Read the model definition and answer for the solid it produces. Units are mm, in the model's axes. Face numbers are marked on the shaded views. A direction names the side the tool comes from. Coordinates: 2 decimals unless noted, no trailing zeros. Write each loop counter-clockwise with the first axis right and the second up, starting at its lowest first coordinate (ties: lowest second). Pieces come first, ordered by that corner, then holes.
(1) Which of the six approach directions +Z, -Z, +X, -X, +Y, -Y give full straight-line access (tool end or side, diameter ignored) to the marked faces 5, 6, 7 and 8?
(2) The part is cut by section A-A, the plane z = 0. Determine the outline of the cut face in (x, y).
(3) The part is cut by section B-B, the plane x = 5. Determine the outline of the cut face in (y, z).
(4) Determine the mould class of the marked faces 1, 2, 3 and 4 for opening direction X: pulls with the +X half, pulls with the -X half, needs draft (parallel to the pull), parting line crosses it, or undercut.
(5) The part is cut by section D-D, the plane z = -2.75. Determine the outline of the cut face in (x, y).
(6) Given pin 1 (1.5 mm diameter, centred on x = 5, z = 0, fed in from -Y) (1 decimal); pin 2 (1.5 mm diameter, centred on x = 9, y = 4, fed in from -Z); pin 3 (2 mm diameter, centred on x = 21, z = 3.5, fed in from -Y); pin 4 (6.5 mm diameter, centred on x = 14, y = 11, fed in from -Z), each flat-ended and moving along its own axis, determine where each tip first touches the part or whether it passes through.
(7) The part is cut by section C-C, the plane y = -0.5. Determine the outline of the cut face in (x, z), and give its area (3 significant figures).
(8) Straight lines are drawn through the part: line 1 along Z through (x, y) = (20, 2.4); line 2 along Z through (x, y) = (20.5, -1.25); line 3 along X through (y, z) = (12, -3). For each, find the intervals that lie inside material, in ascending order.
```python
from build123d import *

# Parameters (mm, degrees)
EXTRUDE_1_DEPTH    = 25
SKETCH_2_R         = 2
EXTRUDE_2_DEPTH    = 6.5
HOLE_WIZARD_M3_1_D = 2.5
CHAMFER_1_SIZE     = 1
CHAMFER_2_SIZE     = 0.5


with BuildPart() as part:
    # 草图1 → 凸台-拉伸1 (new body)
    with BuildSketch(Plane(origin=(0, 0, 0), x_dir=(0, 0, -1), z_dir=(1, 0, 0))):
        Polygon((-7.5, 0), (7.5, 0), (7.5, -3), (10.5, -3), (10.5, 4), (-10.5, 4), (-10.5, -3), (-7.5, -3), align=None)
    extrude(amount=EXTRUDE_1_DEPTH)

    # 草图2 → 凸台-拉伸2 (add, symmetric)
    with BuildSketch(Plane.XY):
        with BuildLine():
            Line((8.5, 12), (8.5, 4))
            Line((8.5, 4), (16.5, 4))
            Line((16.5, 4), (16.5, 12))
            ThreePointArc((16.5, 12), (12.5, 16), (8.5, 12))
        make_face()
        with Locations(Location((12.5, 12, 0), (0, 0, 180))):
            Circle(SKETCH_2_R, mode=Mode.SUBTRACT)
    extrude(amount=EXTRUDE_2_DEPTH, both=True)

    # M3 螺纹孔1 (through all)
    with Locations(Plane(origin=(0, 4, 0), x_dir=(1, 0, 0), z_dir=(0, 1, 0))):
        with Locations((5, 0), (20, 0)):
            Hole(HOLE_WIZARD_M3_1_D / 2)

    # 倒角1
    chamfer_1_edges = [part.edges().sort_by_distance(p)[0] for p in [
        (12.5, 4, 10.5),
        (12.5, 4, -10.5),
    ]]
    chamfer(chamfer_1_edges, length=CHAMFER_1_SIZE)

    # 倒角2
    chamfer_2_edges = [part.edges().sort_by_distance(p)[0] for p in [
        (12.5, -3, 7.5),
        (12.5, -3, 10.5),
        (12.5, -3, -10.5),
        (12.5, -3, -7.5),
    ]]
    chamfer(chamfer_2_edges, length=CHAMFER_2_SIZE)


solid = part.part
```
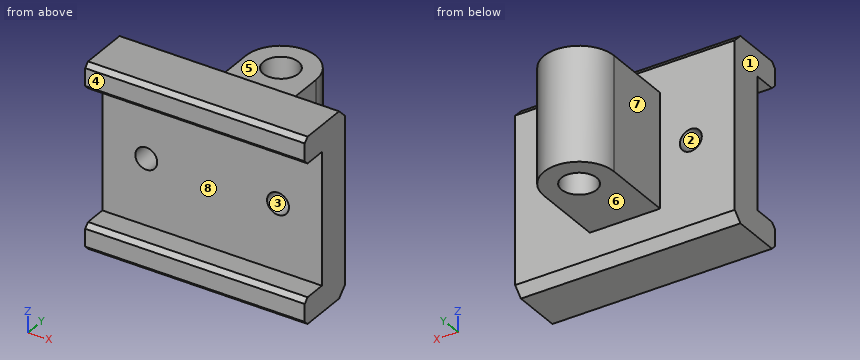
Computed:
1. face 5: +Z, +X, -X, +Y
1. face 6: -Z, +X, -X, +Y
1. face 7: +Z, -Z, -X, +Y
1. face 8: +X, -X, -Y
2. outline: (0, 0) - (3.75, 0) - (3.75, 4) - (0, 4) - close; (6.25, 0) - (18.75, 0) - (18.75, 4) - (16.5, 4) - (16.5, 12) arc R4 ccw to (8.5, 12) - (8.5, 4) - (6.25, 4) - close; (21.25, 0) - (25, 0) - (25, 4) - (21.25, 4) - close; hole circle Ø4 at (12.5, 12)
3. outline: (-3, -10) - (-2.5, -10.5) - (3, -10.5) - (4, -9.5) - (4, -1.25) - (0, -1.25) - (0, -7.5) - (-2.5, -7.5) - (-3, -8) - close; (-3, 8) - (-2.5, 7.5) - (0, 7.5) - (0, 1.25) - (4, 1.25) - (4, 9.5) - (3, 10.5) - (-2.5, 10.5) - (-3, 10) - close
4. face 1: pulls with the -X half
4. face 2: undercut
4. face 3: undercut
4. face 4: needs draft
5. outline: (0, 0) - (25, 0) - (25, 4) - (16.5, 4) - (16.5, 12) arc R4 ccw to (8.5, 12) - (8.5, 4) - (0, 4) - close; hole circle Ø4 at (12.5, 12)
6. pin 1: passes through
6. pin 2: stops at z = -10.25
6. pin 3: stops at y = 0
6. pin 4: stops at z = -6.5
7. outline: (0, -10.5) - (25, -10.5) - (25, -7.5) - (0, -7.5) - close; (0, 7.5) - (25, 7.5) - (25, 10.5) - (0, 10.5) - close
7. area: 150 mm2
8. line 1: z = -10.5 to -1.25, 1.25 to 10.5
8. line 2: z = -10.5 to -7.5, 7.5 to 10.5
8. line 3: x = 8.5 to 10.5, 14.5 to 16.5
